Geometry check sheet. Reference: the model listing, model coordinates, mm. Face numbers are marked on the shaded views. Give positions to 0.01 mm unless a question says otherwise; leave off trailing zeros. Order: outer loops, then holes, each group sorted by start corner. A loop starts at its lowest first (then second) coordinate and runs counter-clockwise, first axis right, second up. Notation, with made-up numbers: M 75.5,5.5 L 82.5,5.5 A35 ccw 82.5,37.5 Z; hole C 51,15.5 d9. An arc over 180 degrees is marked long. Put each result on its own line as item: value. Start each with the question number.
Q1. Section check C-C on y = -4.45. Record the cut outline in (x, z).
Q2. Material ranges on L1, parallel to Z at x = 0, y = -3.55; L2, parallel to Z at x = 0, y = -1.6; L3, parallel to Y at x = 3, z = -5.25 (3 decimals), recorded low to high.
Q3. Go/stop test with flat-tipped pins: pin 1 (2 mm diameter, centred on y = -3.5, z = -2, fed in from +X); pin 2 (2 mm diameter, centred on x = 2, y = -2.5, fed in from -Z); pin 3 (4 mm diameter, centred on x = 1.5, z = 0.5, fed in from -Y). Record where each tip stops, or that it passes through.
Q4. Mould release check, pull along Z, two halves, no side actions. Record for the marked faces 1, 2 and 3: +Z half, -Z half, draft (parallel to the pull), parting line (faces both ways), or undercut.
Q5. Section check D-D on y = -2.5. Record the cut outline in (x, z).
```python
from build123d import *

# Parameters (mm, degrees)
F0_R     = 4.6355
F0_R_2   = 3.429
F1_DEPTH = 3.175
F2_R     = 6.35
F2_R_2   = 4.6355
F2_R_3   = 3.429
F3_DEPTH = 1.905
F4_R     = 0.254


with BuildPart() as f1:
    # F0 (on Front) → F1 (new body)
    with BuildSketch(Plane.XZ):
        Circle(F0_R)
        Circle(F0_R_2, mode=Mode.SUBTRACT)
    extrude(amount=F1_DEPTH)

    # F2 (on face) → F3 (join)
    with BuildSketch(Plane.XZ.offset(3.175)):
        Circle(F2_R)
        Circle(F2_R_2, mode=Mode.SUBTRACT)
        Circle(F2_R_2)
        Circle(F2_R_3, mode=Mode.SUBTRACT)
    extrude(amount=F3_DEPTH)

    # F4
    f4_edges = [f1.edges().sort_by_distance(p)[0] for p in [
        (-6.35, -5.08, 0),
        (-3.429, -5.08, 0),
        (-4.6355, 0, 0),
        (-3.429, 0, 0),
    ]]
    fillet(f4_edges, radius=F4_R)


solid = f1.part
```
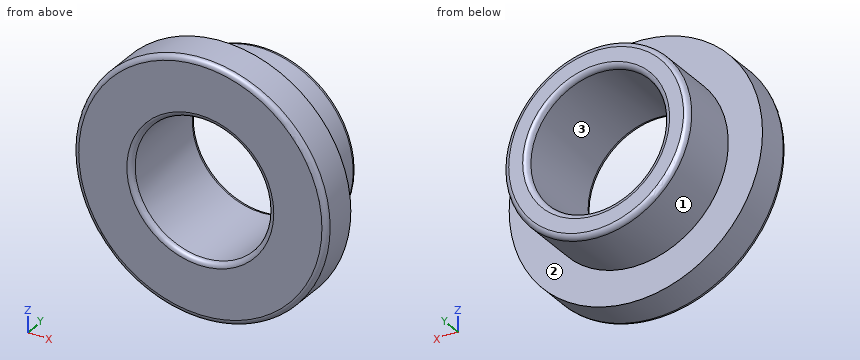
Results found:
1. outline: C 0,0 d12.7; hole C 0,0 d6.86
2. L1: z = -6.35 to -3.43, 3.43 to 6.35
2. L2: z = -4.64 to -3.43, 3.43 to 4.64
2. L3: y = -5.08 to -3.175
3. pin 1: stops at x = 6.27
3. pin 2: stops at z = -6.22
3. pin 3: stops at y = -5.06
4. face 1: parting line
4. face 2: draft
4. face 3: undercut
5. outline: C 0,0 d9.27; hole C 0,0 d6.86
